Autodesk Inventor part; units mm, degrees
ref_plane "YZ Plane" through (0, 0, 0) normal (1, 0, 0) x (0, 1, 0)
ref_plane "XZ Plane" through (0, 0, 0) normal (0, 1, 0) x (-1, 0, 0)
ref_plane "XY Plane" through (0, 0, 0) normal (0, 0, 1) x (1, 0, 0)
sketch "Sketch1" plane through (0, 0, 0) normal (0, 1, 0) x (-1, 0, 0)
  line L0 (16.5, -16.5) -> (-16.5, -16.5)
  line L1 (-16.5, -16.5) -> (-16.5, 16.5)
  line L2 (-16.5, 16.5) -> (16.5, 16.5)
  line L3 (16.5, 16.5) -> (16.5, -16.5)
  point P0 (0, 0)
  point P1 (16.5, 0)
  point P2 (0, -16.5)
  dimension "d0" = 33
  dimension "d1" = 33
extrude "Plate1" add sketch "Sketch1" along normal blind 1.5
sketch "Sketch2" plane through (0, 0, 0) normal (0, 1, 0) x (-1, 0, 0)
  point P0 (0, 0)
  point P1 (0, 0)
hole "Hole1" at (0, 0, 0) direction (0, 1, 0) diameter 6 end through all
sketch "Sketch3" plane through (0, 0, 0) normal (0, 1, 0) x (-1, 0, 0)
  line L0 (0, 0) -> (0, -16.3603)
  point P0 (13, -4)
  point P1 (-13, 4)
  dimension "d10" = 4
  dimension "d11" = 13
  dimension "d12" = 4
  dimension "d13" = 13
hole "Hole2" at (-13, 0, -4) at (13, 0, 4) direction (0, 1, 0) diameter 4.3 end through all
sketch "Sketch4" plane through (0, 0, 0) normal (0, 1, 0) x (-1, 0, 0)
  point P0 (0, 0)
  point P1 (13, -11.5)
  point P2 (-13, 11.5)
  dimension "d21" = 13
  dimension "d22" = 11.5
  dimension "d23" = 11.5
  dimension "d24" = 13
hole "Hole3" at (-13, 0, -11.5) at (13, 0, 11.5) direction (0, 1, 0) diameter 3.6 end through all
equation "\"d8\" = Thickness"
equation "\"d19\" = Thickness"
equation "\"d30\" = Thickness"
equation "\"d32\" = Thickness"
equation "\"BendRadius\" = Thickness"
equation "\"BendReliefWidth\" = Thickness"
equation "\"BendReliefDepth\" = 0.5 * Thickness"
equation "\"CornerReliefSize\" = 4 * Thickness"
equation "\"MinimumRemnant\" = 2 * Thickness"
equation "\"TransitionRadius\" = BendRadius"
equation "\"JacobiRadiusSize\" = BendRadius"
equation "\"GapSize\" = Thickness"
equation "\"d2\" = BendRadius"
properties part number "Luxcan P1"
Read the model definition and answer for the solid it produces. Units are mm, in the model's axes. Round coordinates to 2 decimals unless told otherwise and drop trailing zeros. Write each loop counter-clockwise with the first axis right and the second up, starting at its lowest first coordinate (ties: lowest second). Pieces come first, ordered by that corner, then holes. Notation, with made-up numbers: M -12.75,20.5 L 33.25,20.5 A29 cw 33.25,48.5 Z; hole C 26.25,31.25 d8. An arc over 180 degrees is marked long. Use a Markdown table: item, result.
1) The part is cut by section C-C (x = -13). Write down the section's boundary in (y, z).
Answers follow:
| item | result |
|---|---|
| outline | M 0,-16.5 L 1.5,-16.5 L 1.5,-13.3 L 0,-13.3 Z; M 0,-9.7 L 1.5,-9.7 L 1.5,-6.15 L 0,-6.15 Z; M 0,-1.85 L 1.5,-1.85 L 1.5,16.5 L 0,16.5 Z |
2) The part is cut by section B-B (z = -4). Write down the section's boundary in (x, y).
Answers follow:
| item | result |
|---|---|
| outline | M -16.5,0 L -15.15,0 L -15.15,1.5 L -16.5,1.5 Z; M -10.85,0 L 16.5,0 L 16.5,1.5 L -10.85,1.5 Z |
3) The part is cut by section D-D (y = 1.1). Write down the section's boundary in (x, z), plus the area to 3 significant figures.
Answers follow:
| item | result |
|---|---|
| outline | M -16.5,-16.5 L 16.5,-16.5 L 16.5,16.5 L -16.5,16.5 Z; hole C -13,-4 d4.3; hole C -13,-11.5 d3.6; hole C 0,0 d6; hole C 13,4 d4.3; hole C 13,11.5 d3.6 |
| area | 1,010 mm2 |
4) Straight lines are drawn through the part: line 1 along Z through (x, y) = (13, 1.2); line 2 along Z through (x, y) = (-13, 1.1); line 3 along X through (y, z) = (1.25, 4). For each, find the intervals that lie inside material, in ascending order. Write a range as [from, to].
Answers follow:
| item | result |
|---|---|
| line 1 | z = [-16.5, 1.85], [6.15, 9.7], [13.3, 16.5] |
| line 2 | z = [-16.5, -13.3], [-9.7, -6.15], [-1.85, 16.5] |
| line 3 | x = [-16.5, 10.85], [15.15, 16.5] |
5) The part is cut by section A-A (x = 0). Write down the section's boundary in (y, z).
Answers follow:
| item | result |
|---|---|
| outline | M 0,-16.5 L 1.5,-16.5 L 1.5,-3 L 0,-3 Z; M 0,3 L 1.5,3 L 1.5,16.5 L 0,16.5 Z |
6) For a pull along X with two mould halves and no side action, classify faces 1 (the cylindrical face through (12.92, 0.76, 13.3)), 2 (the flat face through (-16.5, 1, 0)), 3 (the flat face through (0, 1, 16.5)) as pulls with the +X half, pulls with the -X half, needs draft (parallel to the pull), parting line crosses it, or undercut.
Answers follow:
| item | result |
|---|---|
| face 1 | undercut |
| face 2 | pulls with the -X half |
| face 3 | needs draft |
7) A flat-ended cylindrical pin translates along its axis: pin 1 (4.5 mm diameter, centred on x = 13, z = 11.5, fed in from +Y). Find the tip coordinate at first contact, or state that the pin passes through.
Answers follow:
| item | result |
|---|---|
| pin 1 | stops at y = 1.5 |
